```python
from build123d import *

# Parameters (mm, degrees)
SKETCH1_W           = 120
SKETCH1_H           = 36
BOSS_EXTRUDE1_DEPTH = 3.175
SKETCH2_R           = 15
CUT_EXTRUDE1_DEPTH  = 10
SKETCH3_R           = 0.9
CUT_EXTRUDE2_DEPTH  = 10
SKETCH4_R           = 1
CUT_EXTRUDE3_DEPTH  = 10


with BuildPart() as part:
    # Sketch1 → Boss-Extrude1 (new body)
    with BuildSketch(Plane(origin=(0, 0, 0), x_dir=(1, 0, 0), z_dir=(0, 1, 0))):
        Rectangle(SKETCH1_W, SKETCH1_H)
    extrude(amount=BOSS_EXTRUDE1_DEPTH)

    # Sketch2 → Cut-Extrude1 (cut)
    with BuildSketch(Plane(origin=(0, 3.175, 0), x_dir=(1, 0, 0), z_dir=(0, 1, 0))):
        with Locations(Location((0, 0, 0), (0, 0, 270))):
            Circle(SKETCH2_R)
    extrude(amount=-CUT_EXTRUDE1_DEPTH, mode=Mode.SUBTRACT)

    # Sketch3 → Cut-Extrude2 (cut)
    with BuildSketch(Plane(origin=(0, 3.175, 0), x_dir=(1, 0, 0), z_dir=(0, 1, 0))):
        with Locations(Location((12, 12, 0), (0, 0, 270))):
            Circle(SKETCH3_R)
        with Locations(Location((-12, 12, 0), (0, 0, 270))):
            Circle(SKETCH3_R)
        with Locations(Location((12, -12, 0), (0, 0, 270))):
            Circle(SKETCH3_R)
        with Locations(Location((-12, -12, 0), (0, 0, 270))):
            Circle(SKETCH3_R)
    extrude(amount=-CUT_EXTRUDE2_DEPTH, mode=Mode.SUBTRACT)

    # Sketch4 → Cut-Extrude3 (cut)
    with BuildSketch(Plane(origin=(0, 3.175, 0), x_dir=(1, 0, 0), z_dir=(0, 1, 0))):
        with Locations(Location((-50, 10, 0), (0, 0, 270))):
            Circle(SKETCH4_R)
        with Locations(Location((50, 10, 0), (0, 0, 270))):
            Circle(SKETCH4_R)
        with Locations(Location((50, -10, 0), (0, 0, 270))):
            Circle(SKETCH4_R)
        with Locations(Location((-50, -10, 0), (0, 0, 270))):
            Circle(SKETCH4_R)
    extrude(amount=-CUT_EXTRUDE3_DEPTH, mode=Mode.SUBTRACT)


solid = part.part
```
Verification items for the finished model (mm, model axes). Coordinates: 2 decimals unless noted, no trailing zeros. Loops run counter-clockwise (first coordinate to the right, second up) from the corner with the lowest first, then second, coordinate; pieces in that order, holes last. Notation, with made-up numbers: (-2, -0.75) -> (6, -0.75) arc R22 cw to (6, 24.25) -> close; hole circle Ø8 at (5, -36.5). An arc over 180 degrees is marked (long way). Answer in a Markdown table with one row per item. Add a question column.
1. Section check A-A, the plane z = 0. Enter the section's corners in (x, y) (3 decimals).
2. Depth check by flat-ended pin: P1, Ø1.2, axis at x = 50, z = 10, coming from the +Y side. Enter the tip coordinate at first touch or a pass-through.
3. Material ranges on probe 1 along X at (y, z) = (2.5, -12); probe 2 along X at (y, z) = (0.2, 10); probe 3 along X at (y, z) = (1.6, 0), recorded low to high. Write a range as [from, to].
4. Draft check along X on faces 1 (the face through (-60, 2, 0)), 2 (the face through (-1, 2, 18)), 3 (the face through (60, 2, 0)), 4 (the face through (51, 2, -10)). Enter one of: +X half, -X half, draft (parallel to the pull), parting line (faces both ways), or undercut.
5. Section check B-B, the plane x = 0. Enter the section's corners in (y, z) (3 decimals), then the cut area to 4 significant figures.
6. Section check C-C, the plane y = 1.1. Give the number of separate pieces and of enclosed holes in the cut face, then the cut area to 3 significant figures.
Derived:
| question | item | result |
|---|---|---|
| 1 | outline | (-60, 0) -> (-15, 0) -> (-15, 3.175) -> (-60, 3.175) -> close; (15, 0) -> (60, 0) -> (60, 3.175) -> (15, 3.175) -> close |
| 2 | P1 | passes through |
| 3 | probe 1 | x = [-60, -12.9], [-11.1, -9], [9, 11.1], [12.9, 60] |
| 3 | probe 2 | x = [-60, -51], [-49, -11.18], [11.18, 49], [51, 60] |
| 3 | probe 3 | x = [-60, -15], [15, 60] |
| 4 | face 1 | -X half |
| 4 | face 2 | draft |
| 4 | face 3 | +X half |
| 4 | face 4 | undercut |
| 5 | outline | (0, -18) -> (3.175, -18) -> (3.175, -15) -> (0, -15) -> close; (0, 15) -> (3.175, 15) -> (3.175, 18) -> (0, 18) -> close |
| 5 | area | 19.05 mm² |
| 6 | separate pieces | 1 |
| 6 | enclosed holes | 9 |
| 6 | area | 3,590 mm² |
